```python
from build123d import *

# Parameters (mm, degrees)
F1_DEPTH = 25
F2_W     = 49.72059
F2_H     = 76.887056
F3_DEPTH = 3.8
F5_DEPTH = 97.5


with BuildPart() as f1:
    # F0 (on Front) → F1 (new body)
    with BuildSketch(Plane.XZ):
        Polygon((0, 48.325881), (-47.404412, 48.325881), (-47.404412, 38.443528), (-24.860295, 38.443528), (-24.860295, 0), (-24.860295, -38.443528), (-47.404412, -38.443528), (-47.404412, -48.325881), (0, -48.325881), (47.404412, -48.325881), (47.404412, -38.443528), (24.860295, -38.443528), (24.860295, 0), (24.860295, 38.443528), (47.404412, 38.443528), (47.404412, 48.325881), align=None)
    extrude(amount=F1_DEPTH)

    # F2 (on face) → F3 (cut)
    with BuildSketch(Plane.XZ.offset(25)):
        Rectangle(F2_W, F2_H)
    extrude(amount=-F3_DEPTH, mode=Mode.SUBTRACT)

    # F4 (on face) → F5 (cut)
    with BuildSketch(Plane(origin=(0, 0, -48.325881), x_dir=(1, 0, 0), z_dir=(0, 0, -1))):
        with BuildLine():
            Line((-16.650641, 0), (17.627948, 0))
            ThreePointArc((17.627948, 0), (0.488654, 17.139295), (-16.650641, 0))
        make_face()
    extrude(amount=-F5_DEPTH, mode=Mode.SUBTRACT)


solid = f1.part
```
CAD build for the part. Positions are in the model's coordinates, mm. A direction names the side the tool comes from. Give positions to 0.01 mm unless a question says otherwise; leave off trailing zeros. Write each loop counter-clockwise with the first axis right and the second up, starting at its lowest first coordinate (ties: lowest second). Pieces come first, ordered by that corner, then holes. Notation, with made-up numbers: M -3.5,33.25 L 32.5,33.25 A13 cw 32.5,56.25 Z; hole C 54.5,61 d10. An arc over 180 degrees is marked long. Return JSON: item names as keys, results as strings. Group by question number.
(1) Drill centre lines: L1, parallel to Z at x = 37, y = -19.75; L2, parallel to Y at x = 24, z = -5; L3, parallel to X at y = -18.5, z = 3. Where is each one in solid material? Low to high. Write a range as [from, to].
(2) Band-saw the part on A-A (x = 26.5). Give the cut face in (y, z), and give its area (3 significant figures).
(3) Mould opens along X. For faces 1 (the face through (0.866, -17.135, -0.677)), 2 (the face through (47.404, -12, 43)), 3 (the face through (22, 0, 1)) say: pulls with the +X half, pulls with the -X half, needs draft (parallel to the pull), parting line crosses it, or undercut.
(4) Flat gauge pins, fed straight in: pin 1 Ø10 at (x, z) = (-18.5, 27.5) entering from -Y; pin 2 Ø10 at (y, z) = (-22.5, -20.5) entering from +X; pin 3 Ø6 at (y, z) = (-4, 20.5) entering from -X. Where does each tip first touch, or does it go through?
(5) Band-saw the part on B-B (y = -5.5). Give the cut face in (x, z), and give its area (3 significant figures).
(6) Band-saw the part on C-C (z = 5). Give the cut face in (x, y).
(7) 3-axis set-ups, long thin cutter, end or side, ignore diameter. For faces 4 (the face through (1, -23, -38.444)), 5 (the face through (-24.86, -10, 1)), 6 (the face through (0, -21.2, 1)), 7 (the face through (24.86, -10, -1)): which of +Z, -Z, +X, -X, +Y, -Y reach the whole face in a straight line?
(8) Band-saw the part on D-D (y = -19.5). Give the cut face in (x, z).
Entries:
{
 "1": {"L1": "z = [-48.33, -38.44], [38.44, 48.33]", "L2": "y = [-21.2, 0]", "L3": "x = [-24.86, 24.86]"},
 "2": {"outline": "M -25,-48.33 L 0,-48.33 L 0,-38.44 L -25,-38.44 Z; M -25,38.44 L 0,38.44 L 0,48.33 L -25,48.33 Z", "area": "494 mm^2"},
 "3": {"face 1": "undercut", "face 2": "pulls with the +X half", "face 3": "needs draft"},
 "4": {"pin 1": "stops at y = -21.2", "pin 2": "stops at x = 24.86", "pin 3": "stops at x = -24.86"},
 "5": {"outline": "M -47.4,-48.33 L -15.74,-48.33 L -15.74,48.33 L -47.4,48.33 L -47.4,38.44 L -24.86,38.44 L -24.86,-38.44 L -47.4,-38.44 Z; M 16.72,-48.33 L 47.4,-48.33 L 47.4,-38.44 L 24.86,-38.44 L 24.86,38.44 L 47.4,38.44 L 47.4,48.33 L 16.72,48.33 Z", "area": "2,560 mm^2"},
 "6": {"outline": "M -24.86,-21.2 L 24.86,-21.2 L 24.86,0 L 17.63,0 A17.14 cw -16.65,0 L -24.86,0 Z"},
 "7": {"face 4": "-Y", "face 5": "-X, +Y, -Y", "face 6": "+X, -X, -Y", "face 7": "+X, +Y, -Y"},
 "8": {"outline": "M -47.4,-48.33 L 47.4,-48.33 L 47.4,-38.44 L 24.86,-38.44 L 24.86,38.44 L 47.4,38.44 L 47.4,48.33 L -47.4,48.33 L -47.4,38.44 L -24.86,38.44 L -24.86,-38.44 L -47.4,-38.44 Z"}
}
